Geometry check sheet. Reference: the model listing, model coordinates, mm. Face numbers are marked on the shaded views. A direction names the side the tool comes from. Round coordinates to 2 decimals unless told otherwise and drop trailing zeros. Write item = value, one per line.
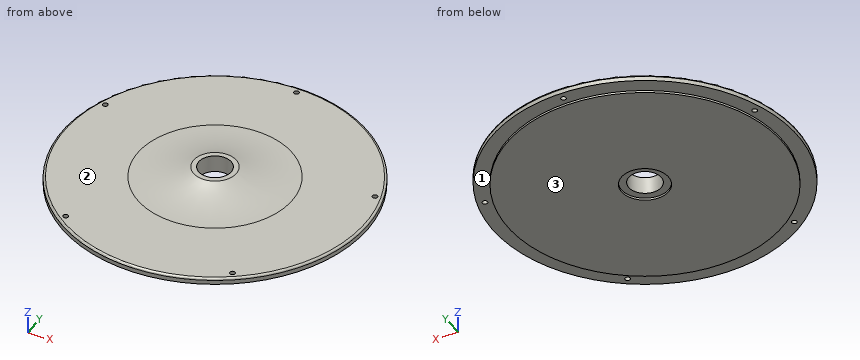
from build123d import *

# Parameters (mm, degrees)
SKETCH2_R           = 81.28
BOSS_EXTRUDE1_DEPTH = 1.27
SKETCH3_R           = 90.17
BOSS_EXTRUDE2_DEPTH = 3.81
SKETCH4_R           = 1.524
CUT_EXTRUDE2_DEPTH  = 128.576541339
CIRPATTERN1_COUNT   = 5
SKETCH14_R          = 12.7
SKETCH14_R_2        = 6.477
BOSS_EXTRUDE3_DEPTH = 6.35
SKETCH23_R          = 13.97
CUT_EXTRUDE3_DEPTH  = 1.27
SKETCH24_R          = 9.652
CUT_EXTRUDE4_DEPTH  = 128.923740564
FILLET1_R           = 88.9
FILLET2_R           = 1.27


with BuildPart() as part:
    # Sketch2 → Boss-Extrude1 (new body)
    with BuildSketch(Plane.XY):
        Circle(SKETCH2_R)
    extrude(amount=-BOSS_EXTRUDE1_DEPTH)

    # Sketch3 → Boss-Extrude2 (add)
    with BuildSketch(Plane.XY):
        with Locations(Location((0, 0, 0), (0, 0, 180))):
            Circle(SKETCH3_R)
    extrude(amount=BOSS_EXTRUDE2_DEPTH)

    # Sketch4 → Cut-Extrude2 (cut, through all)
    with BuildSketch(Plane.XY):
        with Locations(Location((0, 85.725, 0), (0, 0, 180))):
            Circle(SKETCH4_R)
    cut_extrude2 = extrude(amount=CUT_EXTRUDE2_DEPTH, mode=Mode.SUBTRACT)

    # CirPattern1: Cut-Extrude2 ×5 about axis
    cirpattern1_axis = Axis((0, 0, 0), (0, 0, 1))
    for i in range(1, CIRPATTERN1_COUNT):
        add(cut_extrude2.rotate(cirpattern1_axis, i * 360 / CIRPATTERN1_COUNT), mode=Mode.SUBTRACT)

    # Sketch14 → Boss-Extrude3 (add)
    with BuildSketch(Plane.XY.offset(3.81)):
        Circle(SKETCH14_R)
        Circle(SKETCH14_R_2, mode=Mode.SUBTRACT)
    extrude(amount=BOSS_EXTRUDE3_DEPTH)

    # Sketch23 → Cut-Extrude3 (cut)
    with BuildSketch(Plane(origin=(0, 0, -1.27), x_dir=(-1, 0, 0), z_dir=(0, 0, -1))):
        Circle(SKETCH23_R)
    extrude(amount=-CUT_EXTRUDE3_DEPTH, mode=Mode.SUBTRACT)

    # Sketch24 → Cut-Extrude4 (cut, through all)
    with BuildSketch(Plane(origin=(0, 0, 0), x_dir=(-1, 0, 0), z_dir=(0, 0, -1))):
        Circle(SKETCH24_R)
    extrude(amount=-CUT_EXTRUDE4_DEPTH, mode=Mode.SUBTRACT)

    # Fillet1
    # the kernel refuses this fillet: 88.9 mm, written as the material it adds along each edge
    with BuildSketch(Plane(origin=(0, 0, 3.81), x_dir=(1, 0, 0), z_dir=(0, -1, 0))) as fillet1_piece_1:
        with BuildLine():
            CenterArc((45.695567884, 88.9), FILLET1_R, 248.213210702, 21.786789298)
            Line((12.7, 6.35), (12.7, 0))
            Line((12.7, 0), (45.695567884, 0))
        make_face()
    revolve(axis=Axis((0, 0, 3.81), (0, 0, 1)))

    # Fillet2
    fillet2_edges = [part.edges().sort_by_distance(p)[0] for p in [
        (90.17, 0, 3.81),
    ]]
    fillet(fillet2_edges, radius=FILLET2_R)


solid = part.part
(1) Depth check by flat-ended pin: pin 1 Ø4 at (y, z) = (65, 1.5) entering from -X; pin 2 Ø3 at (y, z) = (54.5, 1.5) entering from -X; pin 3 Ø22.5 at (x, y) = (-1.5, -1) entering from -Z. Enter the tip coordinate at first touch or a pass-through.
Result set:
pin_1 = -64.51
pin_2 = -72.95
pin_3 = 0
(2) Material ranges on line 1 along X through (y, z) = (35, 1); line 2 along Z through (x, y) = (-54, 28); line 3 along X through (y, z) = (6, 0.5), recorded low to high. Write a range as from..to.
Result set:
line_1 = -83.1..83.1
line_2 = -1.27..3.81
line_3 = -89.97..-7.56, 7.56..89.97
(3) Tool access check on the marked faces 1, 2 and 3. Record the directions out of +Z, -Z, +X, -X, +Y, -Y that give a thin tool (end or side, any length) a straight path to the whole face; none if there is none.
Result set:
face_1 = -Z
face_2 = +Z
face_3 = -Z, +X, -X, +Y, -Y
